Could you check a few things on this model? Use its own coordinates, in mm. A direction names the side the tool comes from. Round coordinates to 2 decimals unless told otherwise and drop trailing zeros. Write each loop counter-clockwise with the first axis right and the second up, starting at its lowest first coordinate (ties: lowest second). Pieces come first, ordered by that corner, then holes. Notation, with made-up numbers: M 56.25,88.25 L 96.25,88.25 A18 cw 96.25,94.25 Z; hole C -19,7.5 d2. An arc over 180 degrees is marked long. One line per question, with ' | ' between items. Start each with the question number.
```python
from build123d import *

# Parameters (mm, degrees)
CHAFL_N10_SIZE = 0.25
FILLET1_R      = 0.25


with BuildPart() as part:
    # Sketch1 → Revolve1 (revolve)
    with BuildSketch(Plane.XY, mode=Mode.PRIVATE) as revolve1_sk:
        Polygon((-33.87745169, 7.272059531), (-31.87745169, 8), (0, 8), (0, 7), (1.119965147, 7), (1.119965147, 5.380453235), (0, 5.380453235), (-0.979823496, 5.380453235), (-0.979823496, 6), (-33.87745169, 6), align=None)
    revolve(revolve1_sk.sketch.rotate(Axis((0, 0, 0), (-1, 0, 0)), 90), axis=Axis((0, 0, 0), (-1, 0, 0)))

    # Chaflán10
    chafl_n10_edges = [part.edges().sort_by_distance(p)[0] for p in [
        (-33.87745169, 0, 6),
        (-0.979823496, 0, 5.380453235),
        (1.119965147, 0, 5.380453235),
        (1.119965147, 0, 7),
        (0, 0, 7),
    ]]
    chamfer(chafl_n10_edges, length=CHAFL_N10_SIZE)

    # Fillet1
    fillet1_edges = [part.edges().sort_by_distance(p)[0] for p in [
        (-0.979823496, 0, 6),
    ]]
    fillet(fillet1_edges, radius=FILLET1_R)


solid = part.part
```
1. Which directions (+Z, -Z, +X, -X, +Y, -Y) give clear straight access to the entire face, cutting with the end or side of a thin tool? Please do faces 1 (the face through (-17.655, -1.802, -5.723)), 2 (the face through (-15.72, 7.81, 1.73)).
2. If we mould it in two halves opening along Y, with no side actions, what happens to faces 3 (the face through (1.12, 3, 5)), 4 (the face through (0.081, -5.335, 0.7)), 5 (the face through (0.56, 6.21, -3.23))? For each: released by +Y, released by -Y, zero draft, split by the parting line, or undercut.
3. I need wall thicknesses on line 1 along Y through (x, z) = (-19, 0.25); line 2 along Z through (x, y) = (-30, -2.75); line 3 along X through (y, z) = (1.25, 5.5). Which ranges of each line are inside material? Lowest first, please. Write a range as from..to.
4. I'm going to push flat-ended pins straight in: P1, Ø1.5, axis at x = -3.5, y = -2.5, coming from the -Z side; P2, Ø4, axis at x = -19, y = 2, coming from the +Z side; P3, Ø1, axis at x = -30, z = 5, coming from the -Y side; P4, Ø3, axis at x = -22.5, z = -6, coming from the +Y side. Where does each tip first touch, or does it pass through?
5. Suppose I cut it at C-C (x = -5). Write out the boundary of the cut face in (y, z), and give its area (3 significant figures).
Computed:
1) face 1: -X | face 2: +X, -X
2) face 3: zero draft | face 4: undercut | face 5: split by the parting line
3) line 1: y = -8..-5.99, 5.99..8 | line 2: z = -7.51..-5.33, 5.33..7.51 | line 3: x = -0.98..1.12
4) P1: stops at z = -7.81 | P2: stops at z = 8 | P3: stops at y = -6.61 | P4: stops at y = 6.61
5) outline: C 0,0 d16; hole C 0,0 d12 | area: 88.0 mm²
